Autodesk Inventor part; units mm, degrees
ref_plane "YZ Plane" through (0, 0, 0) normal (1, 0, 0) x (0, 1, 0)
ref_plane "XZ Plane" through (0, 0, 0) normal (0, 1, 0) x (-1, 0, 0)
ref_plane "XY Plane" through (0, 0, 0) normal (0, 0, 1) x (1, 0, 0)
sketch "Sketch1" plane through (0, 0, 0) normal (0, 0, 1) x (1, 0, 0)
  line L0 (-70, -70) -> (70, -70)
  line L1 (70, -70) -> (70, 70)
  line L2 (70, 70) -> (-70, 70)
  line L3 (-70, 70) -> (-70, -70)
  line L4 (-70, -70) -> (70, 70) construction
  line L5 (70, -70) -> (-70, 70) construction
  point P0 (0, 0)
  dimension "d0" = 140
  dimension "d1" = 140
extrude "Plate1" add sketch "Sketch1" along normal blind 6
fillet "Corner Round1" radius 20 4 edges at (70, -70, 3) (-70, -70, 3) (-70, 70, 3) (70, 70, 3)
equation "\"d0\" = d1"
equation "\"d2\" = Thickness"
equation "\"BendReliefWidth\" = Thickness"
equation "\"BendReliefDepth\" = 0.5 * Thickness"
equation "\"CornerReliefSize\" = 4 * Thickness"
equation "\"MinimumRemnant\" = 2 * Thickness"
equation "\"TransitionRadius\" = BendRadius"
equation "\"JacobiRadiusSize\" = BendRadius"
equation "\"GapSize\" = Thickness"
properties part number "PNS 1694 leg plate for filter" material "Stainless Steel"
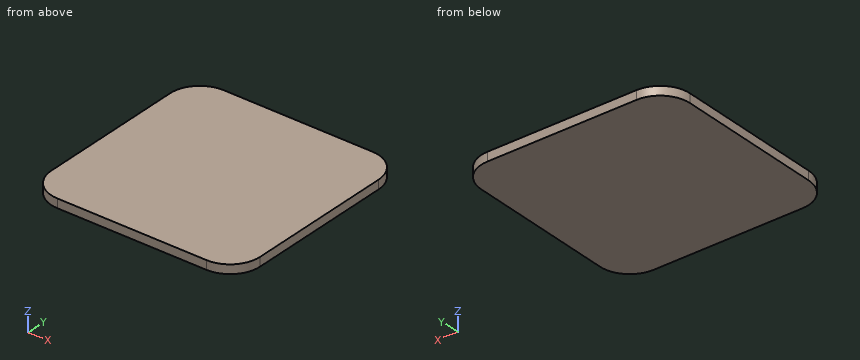
Could you check a few things on this model? Use its own coordinates, in mm. Round coordinates to 2 decimals unless told otherwise and drop trailing zeros. Order: outer loops, then holes, each group sorted by start corner. A loop starts at its lowest first (then second) coordinate and runs counter-clockwise, first axis right, second up. Notation, with made-up numbers: M 72,34 L 118,34 A19 cw 118,50 Z; hole C 35.25,34.5 d2. An arc over 180 degrees is marked long. One line per item, written item: value.
(1) I'm going to push a flat-ended pin straight in: P1, Ø3, axis at x = -54, y = 7.5, coming from the -Z side. Where does the tip first touch, or does it pass through?
Ans:
P1: stops at z = 0
(2) I need wall thicknesses on line 1 along X through (y, z) = (-53.5, 2.9); line 2 along Y through (x, z) = (52.5, 4.05); line 3 along X through (y, z) = (58.5, 5.15). Which ranges of each line are inside material? Lowest first, please. Write a range as from..to.
Ans:
line 1: x = -69.69..69.69
line 2: y = -69.84..69.84
line 3: x = -68.1..68.1
(3) Imagine slicing it at B-B (y = -56.5). Write out the boundary of the cut face in (x, z), and give its area (3 significant figures).
Ans:
outline: M -68.91,0 L 68.91,0 L 68.91,6 L -68.91,6 Z
area: 827 mm^2
(4) Imagine slicing it at A-A (z = 2.05). Write out the boundary of the cut face in (x, y), and give its area (3 significant figures).
Ans:
outline: M -70,-50 A20 ccw -50,-70 L 50,-70 A20 ccw 70,-50 L 70,50 A20 ccw 50,70 L -50,70 A20 ccw -70,50 Z
area: 19,300 mm^2
